Read the model definition and answer for the solid it produces. Units are mm, in the model's axes. Face numbers are marked on the shaded views. A direction names the side the tool comes from. Give positions to 0.01 mm unless a question says otherwise; leave off trailing zeros. Loops run counter-clockwise (first coordinate to the right, second up) from the corner with the lowest first, then second, coordinate; pieces in that order, holes last. Notation, with made-up numbers: (76.25, -13) - (130.25, -13) arc R21 cw to (130.25, 18) - close; hole circle Ø2 at (7, 44). An arc over 180 degrees is marked (long way). Use a Markdown table: item, result. Add a question column.
Item 1: Which of the six approach directions +Z, -Z, +X, -X, +Y, -Y give full straight-line access (tool end or side, diameter ignored) to the marked faces 1, 2 and 3?
Item 2: A cutting plane is placed at A-A (y = -142.5). Determine the outline of the cut face in (x, z), plus the area to 3 significant figures.
Item 3: Consider probe 1 along Y at (x, z) = (7.5, 29); probe 2 along Z at (x, y) = (-1.5, 111.5); probe 3 along Y at (x, z) = (-19.5, -18). Determine where each line is inside the solid, lowest interval first. Write a range as [from, to].
Item 4: A cutting plane is placed at B-B (y = 127.5). Determine the outline of the cut face in (x, z).
Item 5: Each of these flat-tipped pins is pushed along its axis until it touches: P1, Ø5, axis at x = 18.5, y = 24.5, coming from the +Z side; P2, Ø3, axis at x = -23.5, z = 17.5, coming from the +Y side; P3, Ø2, axis at x = 19.5, y = -124, coming from the -Z side; P4, Ø4, axis at x = 8.5, z = -21.5, coming from the +Y side. Where does it stop, or does it pass through?
from build123d import *

# Parameters (mm, degrees)
F0_R      = 32
F1_DEPTH  = 25
F2_R      = 30
F3_DEPTH  = 101
F4_R      = 27.5
F5_DEPTH  = 26
F6_R      = 25
F7_DEPTH  = 11
F8_R      = 30
F9_DEPTH  = 19
F10_R     = 27.5
F11_DEPTH = 19
F12_R     = 24
F13_DEPTH = 110
F14_SIZE  = 1
F15_SIZE  = 1
F16_SIZE  = 1
F17_W     = 1.5
F17_H     = 2.15
F19_SIZE  = 1
F20_SIZE  = 1
F21_SIZE  = 1
F24_DEPTH = 9
F27_DEPTH = 9


with BuildPart() as f1:
    # F0 (on Front) → F1 (new body)
    with BuildSketch(Plane.XZ):
        Circle(F0_R)
    extrude(amount=F1_DEPTH)

    # F2 (on face) → F3 (join)
    with BuildSketch(Plane.XZ.offset(25)):
        Circle(F2_R)
    extrude(amount=F3_DEPTH)

    # F4 (on face) → F5 (join)
    with BuildSketch(Plane.XZ.offset(126)):
        Circle(F4_R)
    extrude(amount=F5_DEPTH)

    # F6 (on face) → F7 (join)
    with BuildSketch(Plane.XZ.offset(152)):
        Circle(F6_R)
    extrude(amount=F7_DEPTH)

    # F8 (on face) → F9 (join)
    with BuildSketch(Plane(origin=(0, 0, 0), x_dir=(-1, 0, 0), z_dir=(0, 1, 0))):
        Circle(F8_R)
    extrude(amount=F9_DEPTH)

    # F10 (on face) → F11 (join)
    with BuildSketch(Plane(origin=(0, 19, 0), x_dir=(-1, 0, 0), z_dir=(0, 1, 0))):
        Circle(F10_R)
    extrude(amount=F11_DEPTH)

    # F12 (on face) → F13 (join)
    with BuildSketch(Plane(origin=(0, 38, 0), x_dir=(-1, 0, 0), z_dir=(0, 1, 0))):
        Circle(F12_R)
    extrude(amount=F13_DEPTH)

    # F14
    f14_edges = [f1.edges().sort_by_distance(p)[0] for p in [
        (24, 148, 0),
    ]]
    chamfer(f14_edges, length=F14_SIZE)

    # F15
    f15_edges = [f1.edges().sort_by_distance(p)[0] for p in [
        (27.5, 38, 0),
    ]]
    chamfer(f15_edges, length=F15_SIZE)

    # F16
    f16_edges = [f1.edges().sort_by_distance(p)[0] for p in [
        (30, 19, 0),
    ]]
    chamfer(f16_edges, length=F16_SIZE)

    # F17 (on Top) → F18 (revolve, cut)
    with BuildSketch(Plane.XY):
        with Locations((29.25, 14.075)):
            Rectangle(F17_W, F17_H)
    revolve(axis=Axis((0, 0, 0), (0, -1, 0)), mode=Mode.SUBTRACT)

    # F19
    f19_edges = [f1.edges().sort_by_distance(p)[0] for p in [
        (-30, -126, 0),
    ]]
    chamfer(f19_edges, length=F19_SIZE)

    # F20
    f20_edges = [f1.edges().sort_by_distance(p)[0] for p in [
        (-27.5, -152, 0),
    ]]
    chamfer(f20_edges, length=F20_SIZE)

    # F21
    f21_edges = [f1.edges().sort_by_distance(p)[0] for p in [
        (-25, -163, 0),
    ]]
    chamfer(f21_edges, length=F21_SIZE)

    # F23 (on offset) → F24 (cut)
    with BuildSketch(Plane.YZ.offset(-24)):
        with BuildLine():
            Line((148, -7), (148, 7))
            Line((148, 7), (86, 7))
            ThreePointArc((86, 7), (79, 0), (86, -7))
            Line((86, -7), (148, -7))
        make_face()
    extrude(amount=F24_DEPTH, mode=Mode.SUBTRACT)

    # F26 (on offset) → F27 (cut)
    with BuildSketch(Plane.YZ.offset(-30)):
        with BuildLine():
            ThreePointArc((-84, -9), (-75, 0), (-84, 9))
            Line((-84, 9), (-116, 9))
            ThreePointArc((-116, 9), (-125, 0), (-116, -9))
            Line((-116, -9), (-84, -9))
        make_face()
    extrude(amount=F27_DEPTH, mode=Mode.SUBTRACT)


solid = f1.part
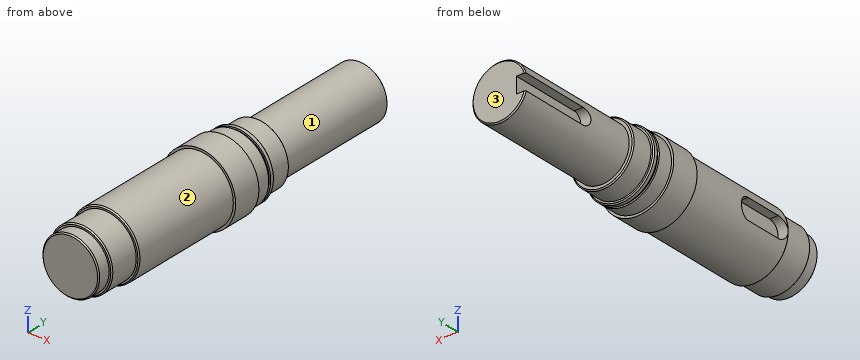
Geometry says:
| question | item | result |
|---|---|---|
| 1 | face 1 | +Y |
| 1 | face 2 | -Y |
| 1 | face 3 | +Z, -Z, +X, -X, +Y |
| 2 | outline | circle Ø55 at (0, 0) |
| 2 | area | 2,380 mm² |
| 3 | probe 1 | [-125.05, 13], [15.15, 18.05] |
| 3 | probe 2 | [-23.95, 23.95] |
| 3 | probe 3 | [-151.96, 37.96] |
| 4 | outline | (-22.96, -7) arc R24 ccw (long way) to (-22.96, 7) - (-15, 7) - (-15, -7) - close |
| 5 | P1 | z = 22.37 |
| 5 | P2 | y = 19 |
| 5 | P3 | z = -23.62 |
| 5 | P4 | y = 148 |
